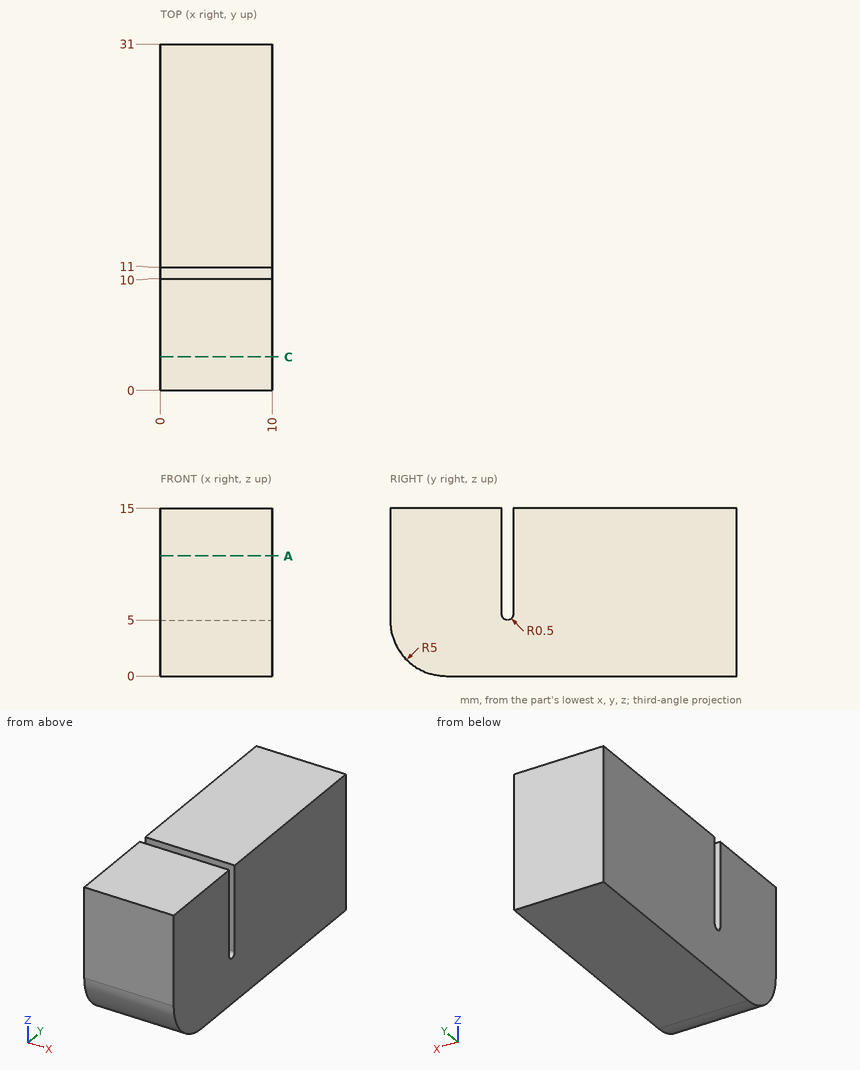
Drawing for the job (mm, zero at the part's lowest x, y, z). Give positions to 0.01 mm unless a question says otherwise; leave off trailing zeros. Order: outer loops, then holes, each group sorted by start corner. A loop starts at its lowest first (then second) coordinate and runs counter-clockwise, first axis right, second up. Notation, with made-up numbers: M 20,-26 L 49,-26 A20 ccw 49,13 Z; hole C 40,6 d9. An arc over 180 degrees is marked long. Use a Markdown table: item, result. Add a question column.
(1) Probe line 1 along Y through (x, z) = (1.5, 5.75); line 2 along Y through (x, z) = (0.5, 1.75); line 3 along Y through (x, z) = (0.75, 0.5). List the from-to ranges inside material, lowest first. Write a range as [from, to].
(2) Drop a flat-ended pin along its axis: P1, Ø3, axis at x = 4.5, z = 5.5, coming from the -Y side. Give the stop position or say it passes through.
(3) Saw through at C-C, the plane y = 3. Give the cut face in (x, z), and give its area (3 significant figures).
(4) Saw through at A-A, the plane z = 10.75. Give the cut face in (x, y), and give its area (3 significant figures).
Answer key:
| question | item | result |
|---|---|---|
| 1 | line 1 | [0, 10], [11, 31] |
| 1 | line 2 | [1.2, 31] |
| 1 | line 3 | [2.82, 31] |
| 2 | P1 | y = 0 |
| 3 | outline | M 0,0.42 L 10,0.42 L 10,15 L 0,15 Z |
| 3 | area | 146 mm^2 |
| 4 | outline | M 0,0 L 10,0 L 10,10 L 0,10 Z; M 0,11 L 10,11 L 10,31 L 0,31 Z |
| 4 | area | 300 mm^2 |
